Build history of the part. All positions in model axes, mm. A direction names the side the tool comes from. Round coordinates to 2 decimals unless told otherwise and drop trailing zeros. Loops run counter-clockwise (first coordinate to the right, second up) from the corner with the lowest first, then second, coordinate; pieces in that order, holes last. Notation, with made-up numbers: (88.5, 60.5) - (135.5, 60.5) arc R27 cw to (135.5, 80.5) - close; hole circle Ø7 at (15.25, 44.25). An arc over 180 degrees is marked (long way). Use one line per item in the form item = value. Start each with the question number.
Q1. Mould opens along Y. For faces 4 (the face through (0, -6, 0)), 5 (the face through (-0.1, -17.3, 0.5)), 6 (the face through (-2.87, 2.64, 0.49)) say: released by +Y, released by -Y, zero draft, split by the parting line, or undercut.
Q2. Pin check, flat tip, straight feed: pin 1 (1.5 mm diameter, centred on x = 2.5, y = -6, fed in from -Z). Stop position of the tip, or through.
Q3. Saw through at D-D (x = 2.5). Give the cut face in (y, z).
Q4. 3-axis set-ups, long thin cutter, end or side, ignore diameter. For faces 1 (the face through (3.36, -9.66, 0.49)), 2 (the face through (-3.347, -9.611, 0.493)), 3 (the face through (0, -6, 1)): which of +Z, -Z, +X, -X, +Y, -Y reach the whole face in a straight line?
Q5. Saw through at C-C (z = 0.5). Give the cut face in (x, y).
Q6. Drill centre lines: line 1 (Y direction, x = 2.75, z = 0.95); line 2 (Y direction, x = 1.5, z = 0.4); line 3 (X direction, y = -10.5, z = 0.15). Where is each one in solid material? Low to high.
Q7. Saw through at B-B (x = 0). Give the cut face in (y, z).
Q8. Saw through at A-A (y = 0). Give the cut face in (x, z), then the cut area to 3 significant figures.
```python
from build123d import *

# Parameters (mm, degrees)
SKETCH_1_R      = 3.9
EXTRUDE_1_DEPTH = 1


with BuildPart() as part:
    # Эскиз1 → Вытянуть1 (new body)
    with BuildSketch(Plane.XY):
        with BuildLine():
            ThreePointArc((3.91695076, -1.774118582), (0, 4.3), (-3.91695076, -1.774118582))
            ThreePointArc((-3.91695076, -1.774118582), (-3.352489907, -3.366100957), (-3.064020566, -5.030375386))
            ThreePointArc((-3.064020566, -5.030375386), (-3, -6.5), (-3.064020566, -7.969624614))
            ThreePointArc((-3.064020566, -7.969624614), (-3.352489907, -9.633899043), (-3.91695076, -11.225881418))
            ThreePointArc((-3.91695076, -11.225881418), (0, -17.3), (3.91695076, -11.225881418))
            ThreePointArc((3.91695076, -11.225881418), (3.352489907, -9.633899043), (3.064020566, -7.969624614))
            ThreePointArc((3.064020566, -7.969624614), (3, -6.5), (3.064020566, -5.030375386))
            ThreePointArc((3.064020566, -5.030375386), (3.352489907, -3.366100957), (3.91695076, -1.774118582))
        make_face()
        Circle(SKETCH_1_R, mode=Mode.SUBTRACT)
        with Locations((0, -13)):
            Circle(SKETCH_1_R, mode=Mode.SUBTRACT)
    extrude(amount=EXTRUDE_1_DEPTH)


solid = part.part
```
Report:
q1.face_4 = zero draft
q1.face_5 = undercut
q1.face_6 = undercut
q2.pin_1 = 0
q3.outline = (-16.5, 0) - (-15.99, 0) - (-15.99, 1) - (-16.5, 1) - close; (-10.01, 0) - (-2.99, 0) - (-2.99, 1) - (-10.01, 1) - close; (2.99, 0) - (3.5, 0) - (3.5, 1) - (2.99, 1) - close
q4.face_1 = +Z, -Z, +X
q4.face_2 = +Z, -Z, -X
q4.face_3 = +Z, +X, -X, +Y, -Y
q5.outline = (-3.92, -11.23) arc R4.3 ccw (long way) to (3.92, -11.23) arc R10 cw to (3.06, -7.97) arc R16.9 cw to (3.06, -5.03) arc R10 cw to (3.92, -1.77) arc R4.3 ccw (long way) to (-3.92, -1.77) arc R10 cw to (-3.06, -5.03) arc R16.9 cw to (-3.06, -7.97) arc R10 cw to start; hole circle Ø7.8 at (0, -13); hole circle Ø7.8 at (0, 0)
q6.line_1 = -16.31 to -15.77, -10.23 to -2.77, 2.77 to 3.31
q6.line_2 = -17.03 to -16.6, -9.4 to -3.6, 3.6 to 4.03
q6.line_3 = -3.62 to -2.99, 2.99 to 3.62
q7.outline = (-17.3, 0) - (-16.9, 0) - (-16.9, 1) - (-17.3, 1) - close; (-9.1, 0) - (-3.9, 0) - (-3.9, 1) - (-9.1, 1) - close; (3.9, 0) - (4.3, 0) - (4.3, 1) - (3.9, 1) - close
q8.outline = (-4.3, 0) - (-3.9, 0) - (-3.9, 1) - (-4.3, 1) - close; (3.9, 0) - (4.3, 0) - (4.3, 1) - (3.9, 1) - close
q8.area = 0.800 mm²
